Verification items for the finished model (mm, model axes). Face numbers are marked on the shaded views. A direction names the side the tool comes from. Coordinates: 2 decimals unless noted, no trailing zeros. Order: outer loops, then holes, each group sorted by start corner. A loop starts at its lowest first (then second) coordinate and runs counter-clockwise, first axis right, second up. Notation, with made-up numbers: (43.25, 69) -> (82.25, 69) arc R19 cw to (82.25, 83) -> close; hole circle Ø1 at (61.5, -17). An arc over 180 degrees is marked (long way). Use CSV: the item, a comma, the result in double quotes. Start each with the question number.
1) Release check for a two-part mould opening along Y. For the marked faces 1, 2 and 3 record: released by +Y, released by -Y, zero draft, split by the parting line, or undercut.
2) Go/stop test with a flat-tipped pin: pin 1 (1 mm diameter, centred on y = 30.5, z = 2.5, fed in from -X). Record where the tip stops, or that it passes through.
3) Sectioned sample at A-A on y = 10. Record the boundary of the cut face in (x, z) (3 decimals), then the cut area to 3 significant figures.
4) Scan lines: line 1 along X through (y, z) = (-9.5, 2.9); line 2 along X through (y, z) = (-4, 3.75); line 3 along X through (y, z) = (5, 5.05). Record each from-to range of solid material in increasing order.
5) Sectioned sample at B-B on y = 0. Record the boundary of the cut face in (x, z), then the cut area to 3 significant figures.
6) Sectioned sample at D-D on y = 16. Record the boundary of the cut face in (x, z), then the cut area to 3 significant figures.
7) Tool access check on the marked faces 4 and 5. Record the directions out of +Z, -Z, +X, -X, +Y, -Y that give a thin tool (end or side, any length) a straight path to the whole face; none if there is none.
Autodesk Inventor part; units mm, degrees
ref_plane "YZ Plane" through (0, 0, 0) normal (1, 0, 0) x (0, 1, 0)
ref_plane "XZ Plane" through (0, 0, 0) normal (0, 1, 0) x (-1, 0, 0)
ref_plane "XY Plane" through (0, 0, 0) normal (0, 0, 1) x (1, 0, 0)
ref_plane "작업 평면1" through (0, 0, 0) normal (0, 0, 1) x (0.3947, 0.9188, 0)
sketch "스케치1" plane through (0, 0, 0) normal (0, 0, 1) x (0.3947, 0.9188, 0)
  point P0 (0, 0)
ref_plane "작업 평면2" through (0, 0, 0) normal (0, 0, 1) x (0.3947, 0.9188, 0)
sketch "스케치2" plane through (0, 0, 0) normal (0, 0, 1) x (0.3947, 0.9188, 0)
  circle A0 centre (0, 0) radius 13.8
  circle A1 centre (0, 0) radius 7.2
  circle A2 centre (0, -11) radius 1.2812
  circle A3 centre (-7.7782, -7.7782) radius 1.2812
  circle A4 centre (-11, 0) radius 1.2812
  circle A5 centre (-7.7782, 7.7782) radius 1.2812
  circle A6 centre (0, 11) radius 1.2812
  circle A7 centre (7.7782, 7.7782) radius 1.2812
  circle A8 centre (11, 0) radius 1.2812
  circle A9 centre (7.7782, -7.7782) radius 1.2812
  line L0 (33.63, -33.63) -> (-32.0037, 32.0037)
  circle A10 centre (0, 0) radius 4.75
  circle A11 centre (0, 0) radius 5.2245
  line L1 (3.6943, -3.6943) -> (-3.6943, 3.6943)
  line L2 (-3.6943, 3.6943) -> (-13.4523, -6.0637)
  line L3 (-13.4523, -6.0637) -> (-6.0637, -13.4523)
  line L4 (-6.0637, -13.4523) -> (3.6943, -3.6943)
  line L5 (9.7581, -9.7581) -> (-9.7581, 9.7581)
  line L6 (-9.7581, 9.7581) -> (18.8336, 38.3497)
  line L7 (18.8336, 38.3497) -> (38.3497, 18.8336)
  line L8 (38.3497, 18.8336) -> (9.7581, -9.7581)
  point P0 (0, 0)
  point P1 (-12.726, -5.3374)
  point P2 (-7.1975, 0.1912)
  point P3 (0.1912, -7.1975)
  point P4 (-5.3374, -12.726)
extrude "돌출1" add sketch "스케치2" along normal blind 6 contours A0 L0 A9 A1 A5 | A0 L6 L7 L8 | L0 A5 A1 L2 A0 | A0 L4 A1 L0 A9
sketch "스케치3" plane through (-27.8029, 32.4408, 6) normal (-0.3706, 0.9288, 0) x (0.9288, 0.3706, 0)
  line L0 (27.6, 6) -> (27.6, 0)
  line L1 (27.6, 6) -> (18.4, 6)
  line L2 (21, 6) -> (6.6, 6)
  line L3 (18.4, 6) -> (9.2, 6)
  line L4 (19.0245, 6) -> (19.0245, 3)
  line L5 (19.0245, 6) -> (19.0245, 0)
  line L6 (9.2, 6) -> (9.2, 3)
  circle A0 centre (19.0245, 3) radius 1.35
  circle A1 centre (9.2, 3) radius 1.35
  point P0 (13.8, 6)
  point P1 (8.5755, 6)
  dimension "d2" = 9.2
  dimension "d3" = 9.2
  dimension "d4" = 3
  dimension "d5" = 3
  dimension "d6" = 2.7
  dimension "d7" = 2.7
extrude "돌출2" cut sketch "스케치3" against normal blind 3
sketch "스케치4" plane through (0, 0, 6) normal (0, 0, 1) x (0.9188, -0.3947, 0)
  line L0 (-23.7306, 29.2101) -> (-21.8214, 31.1192)
  line L1 (-30.6776, 22.2631) -> (-28.7684, 24.1722)
  line L2 (-23.7306, 29.2101) -> (-22.67, 30.2707)
  line L3 (-24.7913, 29.5636) -> (-21.9629, 32.392)
  line L4 (-21.9629, 32.392) -> (-20.5486, 30.9778)
  line L5 (-20.5486, 30.9778) -> (-23.3771, 28.1494)
  line L6 (-23.3771, 28.1494) -> (-24.7913, 29.5636)
  line L7 (-24.7913, 29.5636) -> (-20.5486, 30.9778) construction
  line L8 (-21.9629, 32.392) -> (-23.3771, 28.1494) construction
  line L9 (-30.6776, 22.2631) -> (-29.617, 23.3237)
  line L10 (-31.7383, 22.6166) -> (-28.9099, 25.445)
  line L11 (-28.9099, 25.445) -> (-27.4956, 24.0308)
  line L12 (-27.4956, 24.0308) -> (-30.3241, 21.2024)
  line L13 (-30.3241, 21.2024) -> (-31.7383, 22.6166)
  line L14 (-31.7383, 22.6166) -> (-27.4956, 24.0308) construction
  line L15 (-28.9099, 25.445) -> (-30.3241, 21.2024) construction
  point P0 (0, 0)
  dimension "d10" = 1.5
  dimension "d11" = 4
  dimension "d12" = 2
  dimension "d13" = 1.5
  dimension "d14" = 4
extrude "돌출3" cut sketch "스케치4" against normal blind 3
sketch "스케치5" plane through (0, 0, 0) normal (0, 0, -1) x (-0.9188, 0.3947, 0)
  line L0 (21.8214, 31.1192) -> (23.7306, 29.2101)
  line L1 (28.7684, 24.1722) -> (30.6776, 22.2631)
  line L2 (21.8214, 31.1192) -> (22.8821, 30.0586)
  line L3 (28.7684, 24.1722) -> (29.8291, 23.1116)
  line L4 (23.5892, 27.9373) -> (25.0034, 29.3515)
  line L5 (25.0034, 29.3515) -> (22.175, 32.1799)
  line L6 (22.175, 32.1799) -> (20.7608, 30.7657)
  line L7 (20.7608, 30.7657) -> (23.5892, 27.9373)
  line L8 (23.5892, 27.9373) -> (22.175, 32.1799) construction
  line L9 (25.0034, 29.3515) -> (20.7608, 30.7657) construction
  line L10 (30.5362, 20.9903) -> (31.9504, 22.4045)
  line L11 (31.9504, 22.4045) -> (29.122, 25.2329)
  line L12 (29.122, 25.2329) -> (27.7078, 23.8187)
  line L13 (27.7078, 23.8187) -> (30.5362, 20.9903)
  line L14 (30.5362, 20.9903) -> (29.122, 25.2329) construction
  line L15 (31.9504, 22.4045) -> (27.7078, 23.8187) construction
  point P0 (0, 0)
  dimension "d17" = 1.5
  dimension "d18" = 1.5
  dimension "d19" = 2
  dimension "d20" = 4
  dimension "d21" = 4
extrude "돌출4" cut sketch "스케치5" against normal blind 3
properties part number "_foot_adt"
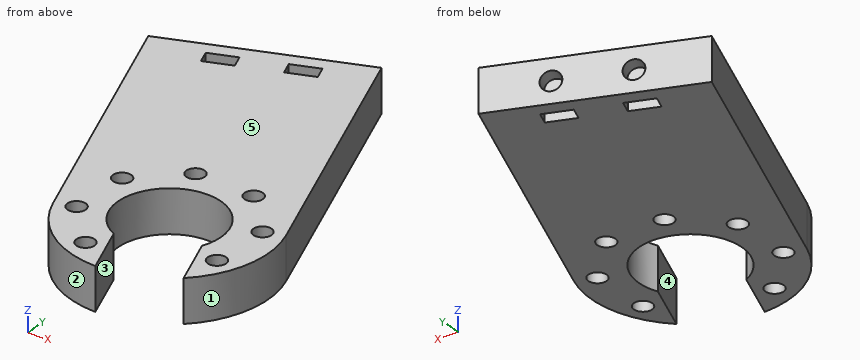
Answers follow:
1,face 1,"split by the parting line"
1,face 2,"released by -Y"
1,face 3,"undercut"
2,pin 1,"stops at x = -27.23"
3,outline,"(-18.848, 0) -> (-5.339, 0) -> (-5.339, 6) -> (-18.848, 6) -> close; (-2.814, 0) -> (3.065, 0) -> (3.065, 6) -> (-2.814, 6) -> close; (5.618, 0) -> (10.868, 0) -> (10.868, 6) -> (5.618, 6) -> close"
3,area,"148 mm²"
4,line 1,"x = -10.01 to -5.47, -3.21 to -1.83, 9.42 to 10.01"
4,line 2,"x = -13.26 to -11.5, -8.94 to -5.99, 7.22 to 8.87, 11.34 to 13.21"
4,line 3,"x = -16.85 to -11.21, -9.01 to -5.18, 5.18 to 9.33, 11.1 to 12.86"
5,outline,"(-14.86, 0) -> (-7.2, 0) -> (-7.2, 6) -> (-14.86, 6) -> close; (7.2, 0) -> (13.8, 0) -> (13.8, 6) -> (7.2, 6) -> close"
5,area,"85.5 mm²"
6,outline,"(-21.24, 0) -> (8.47, 0) -> (8.47, 6) -> (-21.24, 6) -> close"
6,area,"178 mm²"
7,face 4,"+Z, -Z, -Y"
7,face 5,"+Z, +X, -X, +Y, -Y"
